The figure shows three views and two pictorial views of one solid part (mm, origin at its lowest corner). Answer the questions. A direction names the side the tool comes from. Coordinates: 2 decimals unless noted, no trailing zeros. Order: outer loops, then holes, each group sorted by start corner. A loop starts at its lowest first (then second) coordinate and runs counter-clockwise, first axis right, second up. Notation, with made-up numbers: (-37.5, -21) - (-4.5, -21) arc R19 cw to (-4.5, 4) - close; hole circle Ø8 at (37, -3.75). An arc over 180 degrees is marked (long way). Use one line per item in the form item = value.
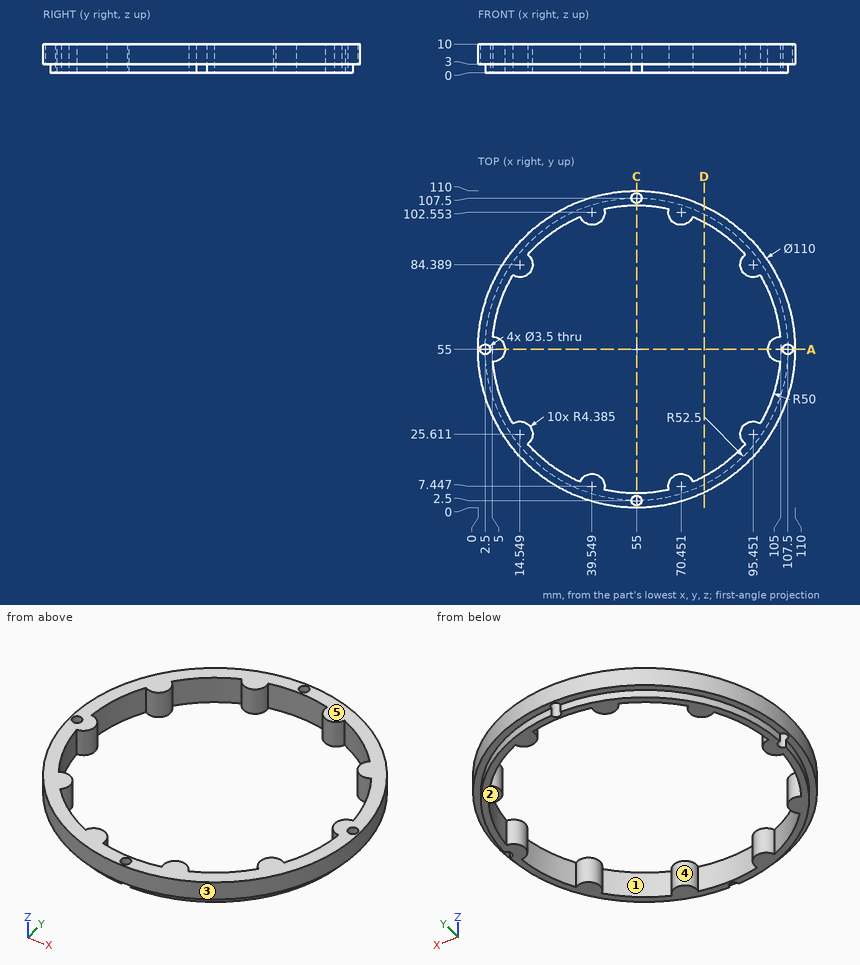
(1) Section C-C, the plane x = 55 is taken. Write down the section's boundary in (y, z).
Answer list:
outline = (0, 3) - (0.75, 3) - (0.75, 10) - (0, 10) - close; (4.25, 0) - (5, 0) - (5, 10) - (4.25, 10) - close; (105, 0) - (105.75, 0) - (105.75, 10) - (105, 10) - close; (109.25, 3) - (110, 3) - (110, 10) - (109.25, 10) - close
(2) The mould has two halves that part along X. Classify the marked faces 3, 4 and 5: +X half, -X half, draft (parallel to the pull), parting line (faces both ways), or undercut.
Answer list:
face_3 = parting line
face_4 = undercut
face_5 = draft
(3) Given pin 1 Ø5.5 at (x, y) = (107.5, 55) entering from -Z; pin 2 Ø1 at (y, z) = (28, 7.5) entering from -X (1 decimal); pin 3 Ø3 at (x, y) = (55, 2.5) entering from -Z; pin 4 Ø3 at (x, z) = (26, 2.5) entering from -Y, each flat-ended and moving along its own axis, determine where each tip first touches the part or whether it passes through.
Answer list:
pin_1 = 0
pin_2 = 6.8
pin_3 = through
pin_4 = 7.42
(4) Section A-A, the plane y = 55 is taken. State how many separate pieces and enclosed holes the cut face has, then the cut area to 3 significant figures.
Answer list:
separate_pieces = 4
enclosed_holes = 0
area = 113 mm2
(5) Straight lines are drawn through the part: L1, parallel to X at y = 56.5, z = 6.5; L2, parallel to X at y = 73.5, z = 5.75 (1 decimal); L3, parallel to Y at x = 84, z = 9.75. For each, find the intervals that lie inside material, in ascending order.
Answer list:
L1 = 0.02 to 1.6, 3.4 to 9.12, 100.88 to 106.6, 108.4 to 109.98
L2 = 3.2 to 8.5, 101.5 to 106.8
L3 = 8.27 to 14.27, 95.73 to 101.73
(6) Which of the six approach directions +Z, -Z, +X, -X, +Y, -Y give full straight-line access (tool end or side, diameter ignored) to the marked faces 1 and 2?
Answer list:
face_1 = +Z, -Z
face_2 = -Z, +X, -X, +Y, -Y
(7) Section D-D, the plane x = 78.5 is taken. Write down the section's boundary in (y, z).
Answer list:
outline = (5.27, 3) - (8.05, 3) - (8.05, 0) - (10.87, 0) - (10.87, 10) - (5.27, 10) - close; (99.13, 0) - (101.95, 0) - (101.95, 3) - (104.73, 3) - (104.73, 10) - (99.13, 10) - close
